Build history of the part. All positions in model axes, mm. A direction names the side the tool comes from. Coordinates: 2 decimals unless noted, no trailing zeros. Loops run counter-clockwise (first coordinate to the right, second up) from the corner with the lowest first, then second, coordinate; pieces in that order, holes last.
Item 1: Flat gauge pins, fed straight in: pin 1 (9 mm diameter, centred on y = 49.25, z = 0, fed in from -X); pin 2 (5 mm diameter, centred on x = -28.28, z = 28.28, fed in from -Y); pin 3 (2 mm diameter, centred on x = 19.5, y = 19.5, fed in from -Z). Where does each tip first touch, or does it go through?
Item 2: Cut at D-D (x = 9). List the corners of the cut face in (y, z), and give its area (3 significant figures).
Item 3: Drill centre lines: line 1 along Y through (x, z) = (23.75, 0); line 2 along Y through (x, z) = (0, 29); line 3 along Y through (x, z) = (-10, -3). Where is each one in solid material? Low to high.
Item 4: Cut at A-A (z = 0). List the corners of the cut face in (x, y), and give its area (3 significant figures).
Item 5: 3-axis set-ups, long thin cutter, end or side, ignore diameter. For faces 4 (the face through (25, 31, 0)), 5 (the face through (-25.62, -8.94, -27.93)), 6 (the face through (17, 31, 0)): which of +Z, -Z, +X, -X, +Y, -Y reach the whole face in a straight line?
Item 6: Cut at B-B (x = 22). List the corners of the cut face in (y, z).
Item 7: Cut at C-C (y = 34.5). List the corners of the cut face in (x, z).
Item 8: Mould opens along Y. For faces 1 (the face through (-21.056, 37.261, 16.827)), 2 (the face through (40, 4, 0)), 3 (the face through (-20.944, 53.217, 0.521)) say: released by +Y, released by -Y, zero draft, split by the parting line, or undercut.
from build123d import *

# Parameters (mm, degrees)
SKETCH1_W           = 80
SKETCH1_H           = 80
BOSS_EXTRUDE1_DEPTH = 8
BOSS_EXTRUDE2_DEPTH = 8
SKETCH5_R           = 4
CUT_EXTRUDE2_DEPTH  = 85
SKETCH6_R           = 15
BOSS_EXTRUDE3_DEPTH = 5
SKETCH7_W           = 80
SKETCH7_H           = 80
SKETCH7_R           = 2.688208694
BOSS_EXTRUDE4_DEPTH = 8
FILLET1_R           = 20
FILLET2_R           = 20


with BuildPart() as part:
    # Sketch1 → Boss-Extrude1 (new body)
    with BuildSketch(Plane(origin=(0, 0, 0), x_dir=(1, 0, 0), z_dir=(0, 1, 0))):
        Rectangle(SKETCH1_W, SKETCH1_H)
    extrude(amount=BOSS_EXTRUDE1_DEPTH)

    # Sketch4 → Boss-Extrude2 (add)
    with BuildSketch(Plane(origin=(-25, 0, 0), x_dir=(0, 0, -1), z_dir=(1, 0, 0))):
        Polygon((-21.161091888, 8), (-12.370414248, 67.35253985), (12.370414248, 67.35253985), (21.161091888, 8), align=None)
    boss_extrude2 = extrude(amount=BOSS_EXTRUDE2_DEPTH)

    # Mirror1: Boss-Extrude2 across plane
    add(boss_extrude2.mirror(Plane(origin=(0, 0, 0), x_dir=(0, 0, 1), z_dir=(1, 0, 0))))

    # Sketch5 → Cut-Extrude2 (cut)
    with BuildSketch(Plane(origin=(25, 0, 0), x_dir=(0, 0, -1), z_dir=(1, 0, 0))):
        with Locations((0, 49.250906007)):
            Circle(SKETCH5_R)
    extrude(amount=-CUT_EXTRUDE2_DEPTH, mode=Mode.SUBTRACT)

    # Sketch6 → Boss-Extrude3 (add)
    with BuildSketch(Plane.XZ):
        with Locations(Location((0, 0, 0), (0, 0, 270))):
            Circle(SKETCH6_R)
    extrude(amount=BOSS_EXTRUDE3_DEPTH)

    # Sketch7 → Boss-Extrude4 (add)
    with BuildSketch(Plane.XZ.offset(5)):
        Rectangle(SKETCH7_W, SKETCH7_H)
        with Locations(Location((-28.284271247, 28.284271247, 0), (0, 0, 270))):
            Circle(SKETCH7_R, mode=Mode.SUBTRACT)
        with Locations(Location((28.284271247, 28.284271247, 0), (0, 0, 270))):
            Circle(SKETCH7_R, mode=Mode.SUBTRACT)
        with Locations(Location((28.284271247, -28.284271247, 0), (0, 0, 270))):
            Circle(SKETCH7_R, mode=Mode.SUBTRACT)
        with Locations(Location((-28.284271247, -28.284271247, 0), (0, 0, 270))):
            Circle(SKETCH7_R, mode=Mode.SUBTRACT)
    extrude(amount=BOSS_EXTRUDE4_DEPTH)

    # Fillet1
    fillet1_edges = [part.edges().sort_by_distance(p)[0] for p in [
        (-40, 4, -40),
    ]]
    fillet(fillet1_edges, radius=FILLET1_R)

    # Fillet2
    fillet2_edges = [part.edges().sort_by_distance(p)[0] for p in [
        (40, 4, 40),
        (-40, 4, 40),
        (40, 4, -40),
    ]]
    fillet(fillet2_edges, radius=FILLET2_R)


solid = part.part
Filled sheet:
1. pin 1: stops at x = -25
1. pin 2: stops at y = 0
1. pin 3: stops at z = -19.61
2. outline: (-13, -40) - (-5, -40) - (-5, -12) - (0, -12) - (0, -40) - (8, -40) - (8, 40) - (0, 40) - (0, 12) - (-5, 12) - (-5, 40) - (-13, 40) - close
2. area: 1,400 mm2
3. line 1: y = -13 to -5, 0 to 45.25, 53.25 to 67.35
3. line 2: y = -13 to -5, 0 to 8
3. line 3: y = -13 to 8
4. outline: (-40, -13) - (40, -13) - (40, -5) - (15, -5) - (15, 0) - (40, 0) - (40, 8) - (25, 8) - (25, 45.25) - (17, 45.25) - (17, 8) - (-17, 8) - (-17, 45.25) - (-25, 45.25) - (-25, 8) - (-40, 8) - (-40, 0) - (-15, 0) - (-15, -5) - (-40, -5) - close; (-25, 53.25) - (-17, 53.25) - (-17, 67.35) - (-25, 67.35) - close; (17, 53.25) - (25, 53.25) - (25, 67.35) - (17, 67.35) - close
4. area: 2,250 mm2
5. face 4: +Z, -Z, +X, +Y
5. face 5: -Y
5. face 6: +Z, -Z, +Y
6. outline: (-13, -40) - (-5, -40) - (-5, 40) - (-13, 40) - close; (0, -39.9) - (8, -39.9) - (8, -21.16) - (67.35, -12.37) - (67.35, 12.37) - (8, 21.16) - (8, 39.9) - (0, 39.9) - close; hole circle Ø8 at (49.25, 0)
7. outline: (-25, -17.24) - (-17, -17.24) - (-17, 17.24) - (-25, 17.24) - close; (17, -17.24) - (25, -17.24) - (25, 17.24) - (17, 17.24) - close
8. face 1: released by +Y
8. face 2: zero draft
8. face 3: undercut
